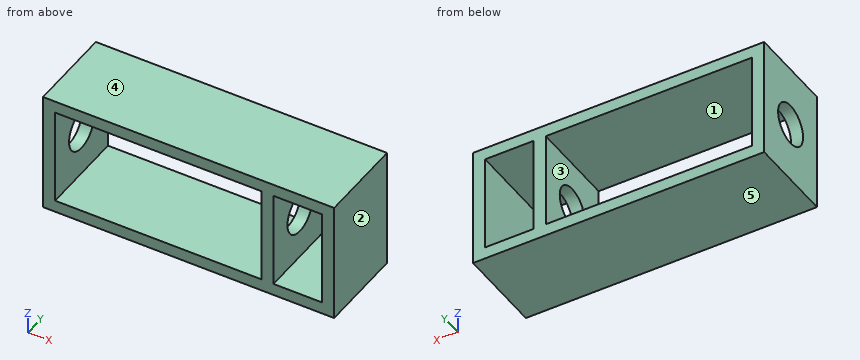
```python
from build123d import *

# Parameters (mm, degrees)
SKETCH1_W           = 60
SKETCH1_H           = 25
SKETCH1_W_2         = 42.5
SKETCH1_H_2         = 20
SKETCH1_W_3         = 10
BOSS_EXTRUDE1_DEPTH = 18
SKETCH3_R           = 4.25
CUT_EXTRUDE1_DEPTH  = 47.5


with BuildPart() as part:
    # Sketch1 → Boss-Extrude1 (new body)
    with BuildSketch(Plane(origin=(0, 0, 0), x_dir=(1, 0, 0), z_dir=(0, 1, 0))):
        with Locations((7.5, 0)):
            Rectangle(SKETCH1_W, SKETCH1_H)
        with Locations((1.25, 0)):
            Rectangle(SKETCH1_W_2, SKETCH1_H_2, mode=Mode.SUBTRACT)
        with Locations((30, 0)):
            Rectangle(SKETCH1_W_3, SKETCH1_H_2, mode=Mode.SUBTRACT)
    extrude(amount=BOSS_EXTRUDE1_DEPTH)

    # Sketch3 → Cut-Extrude1 (cut)
    with BuildSketch(Plane.ZY.offset(22.5)):
        with Locations((0, 9)):
            Circle(SKETCH3_R)
    extrude(amount=-CUT_EXTRUDE1_DEPTH, mode=Mode.SUBTRACT)


solid = part.part
```
Model file for the job. Use its own axes, mm. Face numbers are marked on the shaded views. A direction names the side the tool comes from. Round coordinates to 2 decimals unless told otherwise and drop trailing zeros. Write each loop counter-clockwise with the first axis right and the second up, starting at its lowest first coordinate (ties: lowest second). Pieces come first, ordered by that corner, then holes. Notation, with made-up numbers: (7, 28.5) - (17, 28.5) arc R33 cw to (17, 57.5) - close; hole circle Ø3 at (15.25, 28). An arc over 180 degrees is marked (long way). One line per item, written item: value.
(1) 3-axis set-ups, long thin cutter, end or side, ignore diameter. For the marked faces 1 and 2: which of +Z, -Z, +X, -X, +Y, -Y reach the whole face in a straight line?
Values follow:
face 1: +Y, -Y
face 2: +Z, -Z, +X, +Y, -Y
(2) Cut at D-D, the plane z = 7. Give the cut face in (x, y), plus the area to 3 significant figures.
Values follow:
outline: (-22.5, 0) - (-20, 0) - (-20, 18) - (-22.5, 18) - close; (22.5, 0) - (25, 0) - (25, 18) - (22.5, 18) - close; (35, 0) - (37.5, 0) - (37.5, 18) - (35, 18) - close
area: 135 mm²
(3) Cut at C-C, the plane y = 3.5. Give the cut face in (x, z), plus the area to 3 significant figures.
Values follow:
outline: (-22.5, -12.5) - (37.5, -12.5) - (37.5, 12.5) - (-22.5, 12.5) - close; hole (-20, -10) - (22.5, -10) - (22.5, 10) - (-20, 10) - close; hole (25, -10) - (35, -10) - (35, 10) - (25, 10) - close
area: 450 mm²
(4) Wall check: probe 1 along X at (y, z) = (15.25, 0.5); probe 2 along Z at (x, y) = (-12, 8.25); probe 3 along Y at (x, z) = (23.4, 0). Give the ranges that are in metal, low to high.
Values follow:
probe 1: x = -22.5 to -20, 22.5 to 25, 35 to 37.5
probe 2: z = -12.5 to -10, 10 to 12.5
probe 3: y = 0 to 4.75, 13.25 to 18
(5) Two-plate mould, pull along Z, no slides. Class the marked faces 3, 4 and 5: pulls with the +Z half, pulls with the -Z half, needs draft (parallel to the pull), parting line crosses it, or undercut.
Values follow:
face 3: undercut
face 4: pulls with the +Z half
face 5: pulls with the -Z half
(6) Cut at B-B, the plane x = 19. Give the cut face in (y, z).
Values follow:
outline: (0, -12.5) - (18, -12.5) - (18, -10) - (0, -10) - close; (0, 10) - (18, 10) - (18, 12.5) - (0, 12.5) - close
(7) Cut at A-A, the plane z = 0. Give the cut face in (x, y), plus the area to 3 significant figures.
Values follow:
outline: (-22.5, 0) - (-20, 0) - (-20, 4.75) - (-22.5, 4.75) - close; (-22.5, 13.25) - (-20, 13.25) - (-20, 18) - (-22.5, 18) - close; (22.5, 0) - (25, 0) - (25, 4.75) - (22.5, 4.75) - close; (22.5, 13.25) - (25, 13.25) - (25, 18) - (22.5, 18) - close; (35, 0) - (37.5, 0) - (37.5, 18) - (35, 18) - close
area: 92.5 mm²
(8) Drop a flat-ended pin along its axis: P1, Ø5, axis at y = 9, z = 0, coming from the -X side. Give the stop position or say it passes through.
Values follow:
P1: stops at x = 35
